Check sheet for the modelled part. Datum: model origin and axes. Units: mm. A direction names the side the tool comes from. Coordinates: 2 decimals unless noted, no trailing zeros. Loops run counter-clockwise (first coordinate to the right, second up) from the corner with the lowest first, then second, coordinate; pieces in that order, holes last.
from build123d import *

# Parameters (mm, degrees)
BOSS_EXTRUDE1_DEPTH     = 5.715
CUT_EXTRUDE1_DEPTH      = 6.715
SKETCH4_R               = 4.6355
CUT_EXTRUDE2_DEPTH      = 1
CUT_EXTRUDE2_DEPTH_BACK = 6.715
SKETCH5_W               = 254
SKETCH5_H               = 5.08
CUT_EXTRUDE3_DEPTH      = 6.715
SKETCH6_R               = 4.6355
CUT_EXTRUDE4_DEPTH      = 6.715


with BuildPart() as part:
    # Sketch1 → Boss-Extrude1 (new body)
    with BuildSketch(Plane.XY):
        Polygon((19.05, -63.5), (127, -63.5), (127, -5.715), (132.715, -5.715), (132.715, 6.985), (127, 6.985), (127, 63.5), (-127, 63.5), (-127, 6.985), (-132.715, 6.985), (-132.715, -5.715), (-127, -5.715), (-127, -63.5), (-19.05, -63.5), (-19.05, -114.3), (19.05, -114.3), align=None)
    extrude(amount=BOSS_EXTRUDE1_DEPTH)

    # Sketch2 → Cut-Extrude1 (cut, through all)
    with BuildSketch(Plane.XY.offset(5.715)):
        with BuildLine():
            Line((76.2, -3.175), (-76.2, -3.175))
            ThreePointArc((-76.2, -3.175), (-79.375, 0), (-76.2, 3.175))
            Line((-76.2, 3.175), (76.2, 3.175))
            ThreePointArc((76.2, 3.175), (79.375, 0), (76.2, -3.175))
        make_face()
    extrude(amount=-CUT_EXTRUDE1_DEPTH, mode=Mode.SUBTRACT)

    # Sketch4 → Cut-Extrude2 (cut, two sides)
    with BuildSketch(Plane.XY.offset(5.715)) as cut_extrude2_sk:
        with Locations((0, -50.8)):
            Circle(SKETCH4_R)
    extrude(amount=CUT_EXTRUDE2_DEPTH, mode=Mode.SUBTRACT)
    extrude(cut_extrude2_sk.sketch, amount=-CUT_EXTRUDE2_DEPTH_BACK, mode=Mode.SUBTRACT)

    # Sketch5 → Cut-Extrude3 (cut, through all)
    with BuildSketch(Plane.XY.offset(5.715)):
        with Locations((0, 60.96)):
            Rectangle(SKETCH5_W, SKETCH5_H)
    extrude(amount=-CUT_EXTRUDE3_DEPTH, mode=Mode.SUBTRACT)

    # Sketch6 → Cut-Extrude4 (cut, through all)
    with BuildSketch(Plane.XY.offset(5.715)):
        with Locations((0, -96.52)):
            Circle(SKETCH6_R)
    extrude(amount=-CUT_EXTRUDE4_DEPTH, mode=Mode.SUBTRACT)


solid = part.part
(1) Scan lines: line 1 along Y through (x, z) = (0, 4.1) (1 decimal); line 2 along Y through (x, z) = (58, 3.4) (3 decimals); line 3 along Y through (x, z) = (-13, 2.9) (3 decimals). Record each from-to range of solid material in increasing order.
(2) Section check D-D, the plane x = 0. Enter the section's corners in (y, z) (1 decimal).
(3) Draft check along X on faces 1 (the face through (0, -114.3, 3)), 2 (the face through (-127, 33, 3)), 3 (the face through (-0.603, -91.924, 2.898)). Enter one of: pulls with the +X half, pulls with the -X half, needs draft (parallel to the pull), parting line crosses it, or undercut.
(4) Section check C-C, the plane z = 2.2. Count the separate pieces of the cut face and the enclosed holes in it, plus the area to 3 significant figures.
(5) Section check A-A, the plane x = 30.5. Enter the section's corners in (y, z) (3 decimals).
(6) Set-up check for faces 4 (the face through (-130, -5.715, 3)), 5 (the face through (130, 6.985, 3)), 6 (the face through (72, -63.5, 3)), 7 (the face through (-1, 3.175, 3)): record each of +Z, -Z, +X, -X, +Y, -Y from which the full face is reachable in a straight line by a thin tool's end or side.
(7) Gauge pin test, flat ends, axial feed: P1, Ø3, axis at x = -60, z = 4, coming from the -Y side; P2, Ø5.5, axis at x = 0, y = -50.8, coming from the -Z side; P3, Ø4, axis at x = 70.5, y = -65, coming from the +Z side (3 decimals); P4, Ø3, axis at y = -76.5, z = 3, coming from the -X side. Record the tip position at first contact, or that the pin passes through.
Determined:
1. line 1: y = -114.3 to -101.2, -91.9 to -55.4, -46.2 to -3.2, 3.2 to 58.4
1. line 2: y = -63.5 to -3.175, 3.175 to 58.42
1. line 3: y = -114.3 to -3.175, 3.175 to 58.42
2. outline: (-114.3, 0) - (-101.2, 0) - (-101.2, 5.7) - (-114.3, 5.7) - close; (-91.9, 0) - (-55.4, 0) - (-55.4, 5.7) - (-91.9, 5.7) - close; (-46.2, 0) - (-3.2, 0) - (-3.2, 5.7) - (-46.2, 5.7) - close; (3.2, 0) - (58.4, 0) - (58.4, 5.7) - (3.2, 5.7) - close
3. face 1: needs draft
3. face 2: pulls with the -X half
3. face 3: undercut
4. separate pieces: 1
4. enclosed holes: 3
4. area: 31,900 mm2
5. outline: (-63.5, 0) - (-3.175, 0) - (-3.175, 5.715) - (-63.5, 5.715) - close; (3.175, 0) - (58.42, 0) - (58.42, 5.715) - (3.175, 5.715) - close
6. face 4: +Z, -Z, -X, -Y
6. face 5: +Z, -Z, +X, +Y
6. face 6: +Z, -Z, +X, -Y
6. face 7: +Z, -Z
7. P1: stops at y = -63.5
7. P2: passes through
7. P3: stops at z = 5.715
7. P4: stops at x = -19.05
